Geometry check sheet. Reference: the model listing, model coordinates, mm. Coordinates: 2 decimals unless noted, no trailing zeros. Loops run counter-clockwise (first coordinate to the right, second up) from the corner with the lowest first, then second, coordinate; pieces in that order, holes last.
from build123d import *

# Parameters (mm, degrees)
SKETCH1_R           = 11
BOSS_EXTRUDE1_DEPTH = 10
SKETCH3_R           = 11
CUT_EXTRUDE1_DEPTH  = 10


with BuildPart() as part:
    # Sketch1 → Boss-Extrude1 (new body)
    with BuildSketch(Plane.XY):
        with BuildLine():
            ThreePointArc((-9.87804878, 17.390346526), (-9.770615429, -17.450933332), (19.9888361, 0.668155187))
            ThreePointArc((19.9888361, 0.668155187), (175, 60.751884434), (330.0111639, 0.668155187))
            ThreePointArc((330.0111639, 0.668155187), (359.770615429, -17.450933332), (359.87804878, 17.390346526))
            ThreePointArc((359.87804878, 17.390346526), (175, 118.142256063), (-9.87804878, 17.390346526))
        make_face()
        Circle(SKETCH1_R, mode=Mode.SUBTRACT)
        with Locations((350, 0)):
            Circle(SKETCH1_R, mode=Mode.SUBTRACT)
    extrude(amount=BOSS_EXTRUDE1_DEPTH)

    # Sketch3 → Cut-Extrude1 (cut)
    with BuildSketch(Plane.XY.offset(10)):
        with Locations((175, 90)):
            Circle(SKETCH3_R)
    extrude(amount=-CUT_EXTRUDE1_DEPTH, mode=Mode.SUBTRACT)


solid = part.part
(1) Scan lines: L1, parallel to Y at x = 175, z = 6.5; L2, parallel to X at y = 39, z = 4.25; L3, parallel to X at y = 3, z = 9.25. Record each from-to range of solid material in increasing order.
Findings:
L1: y = 60.75 to 79, 101 to 118.14
L2: x = 6.01 to 77.36, 272.64 to 343.99
L3: x = -19.77 to -10.58, 10.58 to 22.58, 327.42 to 339.42, 360.58 to 369.77
(2) Sectioned sample at C-C on z = 7.5. Record the cut outline in (x, y), and give its area (3 significant figures).
Findings:
outline: (-9.88, 17.39) arc R20 ccw (long way) to (19.99, 0.67) arc R230 cw to (330.01, 0.67) arc R20 ccw (long way) to (359.88, 17.39) arc R220 ccw to start; hole circle Ø22 at (0, 0); hole circle Ø22 at (175, 90); hole circle Ø22 at (350, 0)
area: 20,100 mm2
(3) Sectioned sample at D-D on y = -5. Record the cut outline in (x, z), and give its area (3 significant figures).
Findings:
outline: (-19.36, 0) - (-9.8, 0) - (-9.8, 10) - (-19.36, 10) - close; (9.8, 0) - (19.36, 0) - (19.36, 10) - (9.8, 10) - close; (330.64, 0) - (340.2, 0) - (340.2, 10) - (330.64, 10) - close; (359.8, 0) - (369.36, 0) - (369.36, 10) - (359.8, 10) - close
area: 383 mm2
(4) Gauge pin test, flat ends, axial feed: pin 1 Ø2 at (x, z) = (228, 2) entering from +Y; pin 2 Ø3 at (y, z) = (72.5, 7) entering from -X. Record the tip position at first contact, or that the pin passes through.
Findings:
pin 1: stops at y = 111.91
pin 2: stops at x = 38.91
(5) Draft check along X on faces 1 (the cylindrical face through (359.25, -17.732, 4.93)), 2 (the cylindrical face through (178.07, 118.12, 4.93)), 3 (the flat face through (172, 65, 0)). Enter one of: +X half, -X half, draft (parallel to the pull), parting line (faces both ways), or undercut.
Findings:
face 1: undercut
face 2: parting line
face 3: draft
(6) Sectioned sample at A-A on x = 175. Record the cut outline in (y, z).
Findings:
outline: (60.75, 0) - (79, 0) - (79, 10) - (60.75, 10) - close; (101, 0) - (118.14, 0) - (118.14, 10) - (101, 10) - close
(7) Sectioned sample at B-B on y = 36. Record the cut outline in (x, z).
Findings:
outline: (3.55, 0) - (71.21, 0) - (71.21, 10) - (3.55, 10) - close; (278.79, 0) - (346.45, 0) - (346.45, 10) - (278.79, 10) - close
